```python
from build123d import *

# Parameters (mm, degrees)
F0_R      = 17
F0_R_2    = 14.5
F1_DEPTH  = 4
F2_R      = 14.5
F3_DEPTH  = 1
F4_R      = 3.658597032
F5_DEPTH  = 25
F6_R      = 5.8865262856
F7_DEPTH  = 0.5
F8_R      = 1.1712356188
F9_DEPTH  = 0.5
F10_R     = 2.6152305959
F11_DEPTH = 1.25
F12_R     = 3
F13_DEPTH = 9
F14_R     = 1.525
F15_DEPTH = 8.5


with BuildPart() as f1:
    # F0 (on Front) → F1 (new body)
    with BuildSketch(Plane.XZ):
        Circle(F0_R)
        Circle(F0_R_2, mode=Mode.SUBTRACT)
        Circle(F0_R_2)
    extrude(amount=F1_DEPTH)

    # F2 (on face) → F3 (cut)
    with BuildSketch(Plane.XZ.offset(4)):
        Circle(F2_R)
    extrude(amount=-F3_DEPTH, mode=Mode.SUBTRACT)

    # F4 (on face) → F5 (cut)
    with BuildSketch(Plane.XZ.offset(3)):
        with Locations((-7.0684690372, 7.0684690372)):
            Circle(F4_R)
        with Locations((-9.9963247776, 0)):
            Circle(F4_R)
        with Locations((0, 9.9963247776)):
            Circle(F4_R)
        with Locations((7.0684690372, 7.0684690372)):
            Circle(F4_R)
        with Locations((9.9963247776, 0)):
            Circle(F4_R)
        with Locations((7.0684690372, -7.0684690372)):
            Circle(F4_R)
        with Locations((0, -9.9963247776)):
            Circle(F4_R)
        with Locations((-7.0684690372, -7.0684690372)):
            Circle(F4_R)
    extrude(amount=-F5_DEPTH, mode=Mode.SUBTRACT)

    # F6 (on face) → F7 (join)
    with BuildSketch(Plane.XZ.offset(3)):
        Circle(F6_R)
    extrude(amount=F7_DEPTH)

    # F8 (on face) → F9 (join)
    with BuildSketch(Plane.XZ.offset(3.5)):
        with Locations((-2.9626692521, 2.9626692521)):
            Circle(F8_R)
        with Locations((0, 4.1898470372)):
            Circle(F8_R)
        with Locations((2.9626692521, 2.9626692521)):
            Circle(F8_R)
        with Locations((4.1898470372, 0)):
            Circle(F8_R)
        with Locations((2.9626692521, -2.9626692521)):
            Circle(F8_R)
        with Locations((0, -4.1898470372)):
            Circle(F8_R)
        with Locations((-2.9626692521, -2.9626692521)):
            Circle(F8_R)
        with Locations((-4.1898470372, 0)):
            Circle(F8_R)
    extrude(amount=F9_DEPTH)

    # F10 (on face) → F11 (join)
    with BuildSketch(Plane.XZ.offset(3.5)):
        Circle(F10_R)
    extrude(amount=F11_DEPTH)

    # F12 (on face) → F13 (join)
    with BuildSketch(Plane(origin=(0, 0, 0), x_dir=(-1, 0, 0), z_dir=(0, 1, 0))):
        Circle(F12_R)
    extrude(amount=F13_DEPTH)

    # F14 (on face) → F15 (cut)
    with BuildSketch(Plane(origin=(0, 9, 0), x_dir=(-1, 0, 0), z_dir=(0, 1, 0))):
        Circle(F14_R)
    extrude(amount=-F15_DEPTH, mode=Mode.SUBTRACT)


solid = f1.part
```
Check sheet for the modelled part. Datum: model origin and axes. Units: mm. A direction names the side the tool comes from. Coordinates: 2 decimals unless noted, no trailing zeros. Write each loop counter-clockwise with the first axis right and the second up, starting at its lowest first coordinate (ties: lowest second). Pieces come first, ordered by that corner, then holes. Notation, with made-up numbers: M -6.75,31.25 L 44.25,31.25 A26 ccw 44.25,70.25 Z; hole C 3.5,7.5 d11. An arc over 180 degrees is marked long. Use one line per item in the form item = value.
Item 1: Gauge pin test, flat ends, axial feed: pin 1 Ø11.5 at (x, z) = (0, 10) entering from +Y; pin 2 Ø1.9 at (x, z) = (0.5, -4.5) entering from -Y; pin 3 Ø1.5 at (x, y) = (6, 1.5) entering from -Z; pin 4 Ø2 at (x, y) = (-3, -2) entering from +Z. Record the tip position at first contact, or that the pin passes through.
Answer below:
pin_1 = 0
pin_2 = -4
pin_3 = through
pin_4 = 16.88
Item 2: Release check for a two-part mould opening along X. For faces 4 (the face through (-13.65, -1.52, 0.16)), 5 (the face through (13, -4, 8)), 6 (the face through (3, 4, 0)), 7 (the face through (3, -3.5, -1)) record: pulls with the +X half, pulls with the -X half, needs draft (parallel to the pull), parting line crosses it, or undercut.
Answer below:
face_4 = undercut
face_5 = needs draft
face_6 = parting line crosses it
face_7 = undercut
Item 3: Sectioned sample at A-A, the plane z = 8. Record the cut outline in (x, y), and give its area (3 significant figures).
Answer below:
outline = M -15,-4 L -12.09,-4 L -12.09,-3 L -10.61,-3 L -10.61,0 L -15,0 Z; M -3.53,-3 L -3.07,-3 L -3.07,0 L -3.53,0 Z; M 3.07,-3 L 3.53,-3 L 3.53,0 L 3.07,0 Z; M 10.61,-3 L 12.09,-3 L 12.09,-4 L 15,-4 L 15,0 L 10.61,0 Z
area = 35.0 mm^2
Item 4: Material ranges on L1, parallel to Z at x = 0, y = -3.4; L2, parallel to Z at x = 0, y = 7 (3 decimals); L3, parallel to Y at x = 11, z = -5.5, recorded low to high. Write a range as from..to.
Answer below:
L1 = -17..-14.5, -5.89..5.89, 14.5..17
L2 = -3..-1.525, 1.525..3
L3 = -3..0
Item 5: Sectioned sample at D-D, the plane x = -7.5. Record the cut outline in (y, z), and give its area (3 significant figures).
Answer below:
outline = M -4,-15.26 L 0,-15.26 L 0,-10.7 L -3,-10.7 L -3,-12.41 L -4,-12.41 Z; M -4,12.41 L -3,12.41 L -3,10.7 L 0,10.7 L 0,15.26 L -4,15.26 Z; M -3,-3.44 L 0,-3.44 L 0,-2.67 L -3,-2.67 Z; M -3,2.67 L 0,2.67 L 0,3.44 L -3,3.44 Z
area = 37.6 mm^2
Item 6: Set-up check for faces 1 (the face through (-3, -4, 3)), 2 (the face through (-5.12, -3.75, -0.71)), 3 (the face through (0, -4, 4)): record each of +Z, -Z, +X, -X, +Y, -Y from which the full face is reachable in a straight line by a thin tool's end or side.
Answer below:
face_1 = +Z, -X, -Y
face_2 = -Y
face_3 = +Z, +X, -X, -Y
Item 7: Sectioned sample at B-B, the plane y = -2.5. State how many separate pieces and enclosed holes the cut face has, and give its area (3 significant figures).
Answer below:
separate_pieces = 1
enclosed_holes = 8
area = 572 mm^2
